Model file for the job. Use its own axes, mm. Coordinates: 2 decimals unless noted, no trailing zeros. Order: outer loops, then holes, each group sorted by start corner. A loop starts at its lowest first (then second) coordinate and runs counter-clockwise, first axis right, second up. Notation, with made-up numbers: (34, -26) -> (93, -26) arc R15 ccw to (93, -2) -> close; hole circle Ø2 at (67, 60.5). An arc over 180 degrees is marked (long way). Use CSV: the item, a comma, the result in double quotes. Start each with the question number.
(1) Probe L1, parallel to X at y = 47, z = 0.5; L2, parallel to Z at x = 10, y = 59; L3, parallel to X at y = 13, z = -2. List the from-to ranges inside material, lowest first.
(2) Cut at B-B on z = -8. Write the cut outline in (x, y).
(3) Pin check, flat tips, straight feed: pin 1 Ø3 at (y, z) = (50.5, -7) entering from +X; pin 2 Ø5 at (y, z) = (18, -5.5) entering from +X. Stop position of each tip, or through.
(4) Cut at A-A on z = 7.5. Write the cut outline in (x, y).
```python
from build123d import *

# Parameters (mm, degrees)
BOSS_EXTRUDE1_DEPTH = 66


with BuildPart() as part:
    # Sketch1 → Boss-Extrude1 (new body)
    with BuildSketch(Plane(origin=(0, 0, 0), x_dir=(1, 0, 0), z_dir=(0, 1, 0))):
        with BuildLine():
            ThreePointArc((0.496605757, 9.487011264), (6.890854617, 6.539581229), (9.5, 0))
            Line((9.5, 0), (9.5, 9))
            add(Edge.make_bspline(
                [(0.496605757, 9.487011264), (3.439590397, 9.392632679), (6.469795198, 9), (9.5, 9)],
                knots=[0.303368247, 0.303368247, 0.303368247, 0.303368247, 0.5, 0.5, 0.5, 0.5], degree=3))
        make_face()
        with BuildLine():
            ThreePointArc((0.496605757, -9.487011264), (6.890854617, -6.539581229), (9.5, 0))
            ThreePointArc((9.5, 0), (6.890854617, 6.539581229), (0.496605757, 9.487011264))
            add(Edge.make_bspline(
                [(0, 9.5), (0.165247966, 9.496699631), (0.330788419, 9.492328861), (0.496605757, 9.487011264)],
                knots=[0.292289374, 0.292289374, 0.292289374, 0.292289374, 0.303368247, 0.303368247, 0.303368247, 0.303368247], degree=3))
            ThreePointArc((0, 9.5), (-9.5, 0), (0, -9.5))
            add(Edge.make_bspline(
                [(0, -9.5), (0.165247966, -9.496699631), (0.330788419, -9.492328861), (0.496605757, -9.487011264)],
                knots=[0.292289374, 0.292289374, 0.292289374, 0.292289374, 0.303368247, 0.303368247, 0.303368247, 0.303368247], degree=3))
        make_face()
        with BuildLine():
            ThreePointArc((18.503394243, -9.487011264), (12.109145383, -6.539581229), (9.5, 0))
            ThreePointArc((9.5, 0), (6.890854617, -6.539581229), (0.496605757, -9.487011264))
            add(Edge.make_bspline(
                [(0.496605757, -9.487011264), (3.439590397, -9.392632679), (9.5, -8.607367321), (15.560409603, -9.392632679), (18.503394243, -9.487011264)],
                knots=[0.303368247, 0.303368247, 0.303368247, 0.303368247, 0.5, 0.696631753, 0.696631753, 0.696631753, 0.696631753], degree=3))
        make_face()
        with BuildLine():
            Line((9.5, 9), (9.5, 0))
            ThreePointArc((9.5, 0), (12.109145383, 6.539581229), (18.503394243, 9.487011264))
            add(Edge.make_bspline(
                [(9.5, 9), (12.530204802, 9), (15.560409603, 9.392632679), (18.503394243, 9.487011264)],
                knots=[0.5, 0.5, 0.5, 0.5, 0.696631753, 0.696631753, 0.696631753, 0.696631753], degree=3))
        make_face()
        with BuildLine():
            ThreePointArc((18.503394243, 9.487011264), (12.109145383, 6.539581229), (9.5, 0))
            ThreePointArc((9.5, 0), (12.109145383, -6.539581229), (18.503394243, -9.487011264))
            add(Edge.make_bspline(
                [(18.503394243, -9.487011264), (18.669211581, -9.492328861), (18.834752034, -9.496699631), (19, -9.5)],
                knots=[0.696631753, 0.696631753, 0.696631753, 0.696631753, 0.707710626, 0.707710626, 0.707710626, 0.707710626], degree=3))
            ThreePointArc((19, -9.5), (25.717514421, -6.717514421), (28.5, 0))
            ThreePointArc((28.5, 0), (25.717514421, 6.717514421), (19, 9.5))
            add(Edge.make_bspline(
                [(18.503394243, 9.487011264), (18.669211581, 9.492328861), (18.834752034, 9.496699631), (19, 9.5)],
                knots=[0.696631753, 0.696631753, 0.696631753, 0.696631753, 0.707710626, 0.707710626, 0.707710626, 0.707710626], degree=3))
        make_face()
    extrude(amount=BOSS_EXTRUDE1_DEPTH)


solid = part.part
```
Outcome:
1,L1,"-9.49 to 28.49"
1,L2,"-9 to 9"
1,L3,"-9.29 to 28.29"
2,outline,"(-5.12, 0) -> (24.12, 0) -> (24.12, 66) -> (-5.12, 66) -> close"
3,pin 1,"x = 26.75"
3,pin 2,"x = 28.01"
4,outline,"(-5.83, 0) -> (24.83, 0) -> (24.83, 66) -> (-5.83, 66) -> close"
